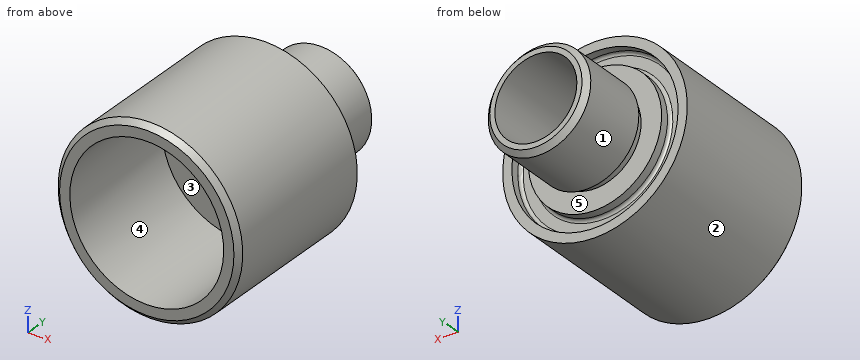
```python
from build123d import *

# Parameters (mm, degrees)
SKETCH_1_R          = 9
EXTRUDE_1_DEPTH     = 16
SKETCH_2_R          = 7.5
CUT_EXTRUDE_1_DEPTH = 12.5
SKETCH_4_R          = 4.5
EXTRUDE_2_DEPTH     = 1
SKETCH_5_R          = 5
EXTRUDE_3_DEPTH     = 7
SKETCH_6_R          = 8.1
SKETCH_6_R_2        = 6.5
CUT_EXTRUDE_2_DEPTH = 1.1
CHAMFER_1_SIZE      = 0.5
FILLET_1_R          = 0.3
SKETCH_15_R         = 4
CUT_EXTRUDE_4_DEPTH = 11.5
CHAMFER_4_SIZE      = 0.5
CHAMFER_5_SIZE      = 0.5


with BuildPart() as part:
    # 草图1 → 凸台-拉伸1 (new body)
    with BuildSketch(Plane(origin=(0, 0, 0), x_dir=(1, 0, 0), z_dir=(0, 1, 0))):
        with Locations(Location((0, 0, 0), (0, 0, 270))):
            Circle(SKETCH_1_R)
    extrude(amount=EXTRUDE_1_DEPTH)

    # 草图2 → 切除-拉伸1 (cut)
    with BuildSketch(Plane.XZ):
        with Locations(Location((0, 0, 0), (0, 0, 270))):
            Circle(SKETCH_2_R)
    extrude(amount=-CUT_EXTRUDE_1_DEPTH, mode=Mode.SUBTRACT)

    # 草图4 → 凸台-拉伸2 (add)
    with BuildSketch(Plane(origin=(0, 16, 0), x_dir=(1, 0, 0), z_dir=(0, 1, 0))):
        with Locations(Location((0, 0, 0), (0, 0, 270))):
            Circle(SKETCH_4_R)
    extrude(amount=EXTRUDE_2_DEPTH)

    # 草图5 → 凸台-拉伸3 (add)
    with BuildSketch(Plane(origin=(0, 17, 0), x_dir=(1, 0, 0), z_dir=(0, 1, 0))):
        with Locations(Location((0, 0, 0), (0, 0, 270))):
            Circle(SKETCH_5_R)
    extrude(amount=EXTRUDE_3_DEPTH)

    # 草图6 → 切除-拉伸2 (cut)
    with BuildSketch(Plane(origin=(0, 16, 0), x_dir=(1, 0, 0), z_dir=(0, 1, 0))):
        with Locations(Location((0, 0, 0), (0, 0, 270))):
            Circle(SKETCH_6_R)
        with Locations(Location((0, 0, 0), (0, 0, 270))):
            Circle(SKETCH_6_R_2, mode=Mode.SUBTRACT)
    extrude(amount=-CUT_EXTRUDE_2_DEPTH, mode=Mode.SUBTRACT)

    # 倒角1
    chamfer_1_edges = [part.edges().sort_by_distance(p)[0] for p in [
        (0, 24, -5),
    ]]
    chamfer(chamfer_1_edges, length=CHAMFER_1_SIZE)

    # 圆角1
    fillet_1_edges = [part.edges().sort_by_distance(p)[0] for p in [
        (0, 14.9, -8.1),
        (0, 14.9, -6.5),
    ]]
    fillet(fillet_1_edges, radius=FILLET_1_R)

    # 草图15 → 切除-拉伸4 (cut)
    with BuildSketch(Plane(origin=(0, 24, 0), x_dir=(1, 0, 0), z_dir=(0, 1, 0))):
        with Locations(Location((0, 0, 0), (0, 0, 270))):
            Circle(SKETCH_15_R)
    extrude(amount=-CUT_EXTRUDE_4_DEPTH, mode=Mode.SUBTRACT)

    # 倒角4
    chamfer_4_edges = [part.edges().sort_by_distance(p)[0] for p in [
        (0, 12.5, -4),
    ]]
    chamfer(chamfer_4_edges, length=CHAMFER_4_SIZE)

    # 倒角5
    chamfer_5_edges = [part.edges().sort_by_distance(p)[0] for p in [
        (0, 0, -9),
    ]]
    chamfer(chamfer_5_edges, length=CHAMFER_5_SIZE)


solid = part.part
```
The listing builds one solid part. Answer for the finished solid, in the listing's coordinates (mm). Face numbers are marked on the shaded views. A direction names the side the tool comes from. Give positions to 0.01 mm unless a question says otherwise; leave off trailing zeros. Order: outer loops, then holes, each group sorted by start corner. A loop starts at its lowest first (then second) coordinate and runs counter-clockwise, first axis right, second up. Notation, with made-up numbers: (-25.75, -29.5) -> (23.25, -29.5) arc R16 cw to (23.25, -15.5) -> close; hole circle Ø6 at (-18.5, 21). An arc over 180 degrees is marked (long way). Answer as a JSON object with one key per item and string values. Group by question number.
Item 1: The part is cut by section A-A on y = 10.25. Write down the section's boundary in (x, z), and give its area (3 significant figures).
Item 2: A tool of negligible diameter and unlimited length cuts with its end or side. For the marked faces 1 and 2, from which of +Z, -Z, +X, -X, +Y, -Y can it reach the whole face along a straight path? Write none if from no direction.
Item 3: Determine the mould class of the marked faces 3, 4 and 5 for opening direction Y: pulls with the +Y half, pulls with the -Y half, needs draft (parallel to the pull), parting line crosses it, or undercut.
Item 4: Flat-ended cylindrical pins translate along their axes: pin 1 (3 mm diameter, centred on x = -5.5, y = 13.5, fed in from +Z); pin 2 (9.5 mm diameter, centred on x = 0, z = 0, fed in from -Y); pin 3 (2 mm diameter, centred on x = 3, y = 8, fed in from +Z); pin 4 (6.5 mm diameter, centred on x = 0, z = 0, fed in from -Y). Find the tip coordinate at first contact, or state that the pin passes through.
Item 5: Consider L1, parallel to X at y = 15.45, z = 0; L2, parallel to X at y = 18.25, z = 0; L3, parallel to X at y = 5, z = 0. Determine where each line is inside the solid, lowest interval first. Write a range as from..to.
Result set:
{
 "1": {"outline": "circle Ø18 at (0, 0); hole circle Ø15 at (0, 0)", "area": "77.8 mm²"},
 "2": {"face 1": "+Y", "face 2": "+Y, -Y"},
 "3": {"face 3": "pulls with the -Y half", "face 4": "needs draft", "face 5": "undercut"},
 "4": {"pin 1": "z = 8.06", "pin 2": "y = 12.5", "pin 3": "z = 8.77", "pin 4": "through"},
 "5": {"L1": "-9..-8.1, -6.5..-4, 4..6.5, 8.1..9", "L2": "-5..-4, 4..5", "L3": "-9..-7.5, 7.5..9"}
}
